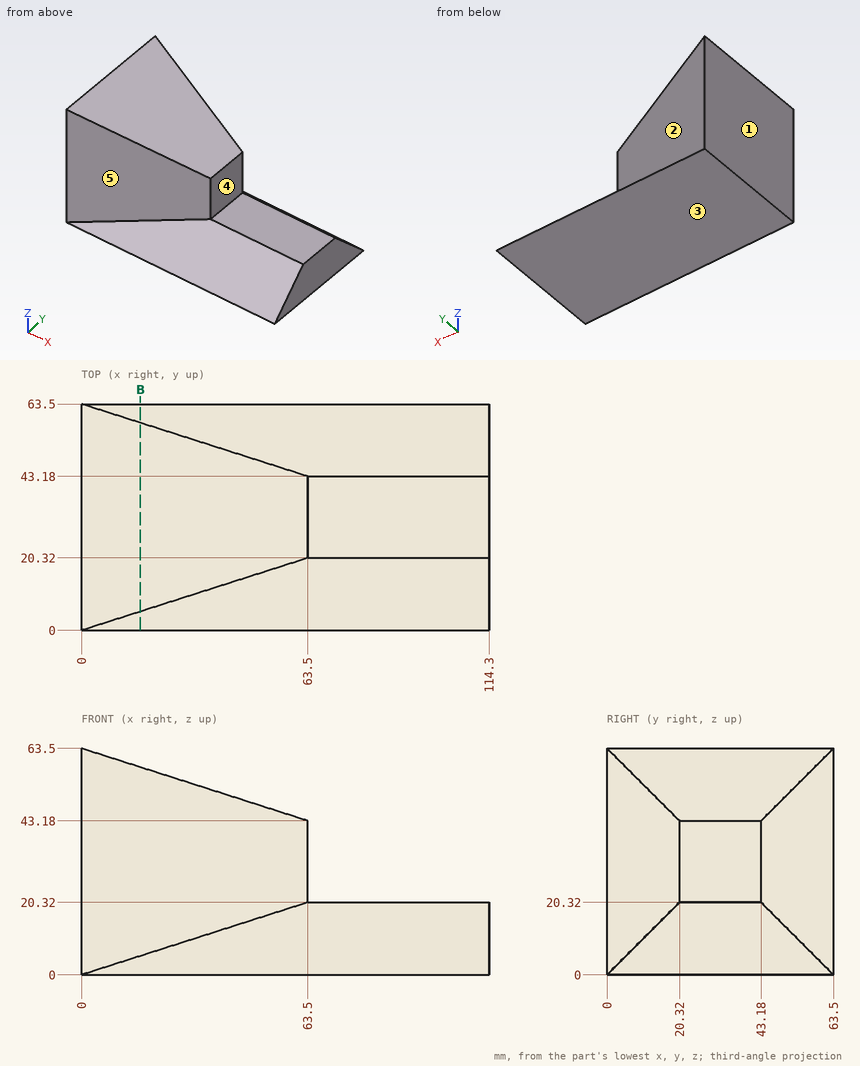
Here's the drawing with two shaded views (mm, measured from the low corner). I have some questions. A direction names the side the tool comes from. Coordinates: 2 decimals unless noted, no trailing zeros. Loops run counter-clockwise (first coordinate to the right, second up) from the corner with the lowest first, then second, coordinate; pieces in that order, holes last. Notation, with made-up numbers: M -12,80 L 46,80 A30 ccw 46,106 Z; hole C 89.25,-12.75 d5. An arc over 180 degrees is marked long. Return JSON: item names as keys, results as strings. Group by question number.
Item 1: If I drill on L1, parallel to Z at x = 91, y = 23; L2, parallel to X at y = 20.5, z = 26; L3, parallel to Z at x = 30, y = 30.5, over which ranges is the centre line in solid material (lowest first)? Write a range as from..to.
Item 2: I'm going to push flat-ended pins straight in: pin 1 Ø6 at (x, z) = (66, 33) entering from +Y; pin 2 Ø8 at (y, z) = (24.5, 28) entering from +X; pin 3 Ø10 at (x, z) = (42.5, 11.5) entering from +Y. Where does each tip first touch, or does it pass through?
Item 3: On a 3-axis mill with a long thin cutter (end or side, diameter ignored), from which of +Z, -Z, +X, -X, +Y, -Y can I reach the whole of each face in a straight line? I mean the marked faces 1, 2, 3, 4 and 5. Say none if no direction works.
Item 4: Imagine slicing it at B-B (x = 16.5). Please give me the cut outline in (y, z), and give its area (3 significant figures).
Verdict:
{
 "1": {"L1": "z = 0..20.32", "L2": "x = 0..63.5", "L3": "z = 0..53.9"},
 "2": {"pin 1": "stops at y = 43.34", "pin 2": "stops at x = 63.5", "pin 3": "stops at y = 57"},
 "3": {"face 1": "+Z, -Z, -X, +Y, -Y", "face 2": "+Z, +X, +Y", "face 3": "-Z, +X, -X, +Y, -Y", "face 4": "+Z, +X, +Y, -Y", "face 5": "+Z, +X, -Y"},
 "4": {"outline": "M 0,0 L 63.5,0 L 58.22,5.28 L 58.22,58.22 L 5.28,58.22 L 5.28,5.28 Z", "area": "3,110 mm^2"}
}
